Read the model definition and answer for the solid it produces. Units are mm, in the model's axes. A direction names the side the tool comes from. Coordinates: 2 decimals unless noted, no trailing zeros. Loops run counter-clockwise (first coordinate to the right, second up) from the corner with the lowest first, then second, coordinate; pieces in that order, holes last. Notation, with made-up numbers: M 41.25,57.25 L 98.25,57.25 A23 ccw 98.25,72.25 Z; hole C 54,63.25 d8. An arc over 180 degrees is marked long. One line per item, written item: value. Start each with the question number.
1. Flat-ended cylindrical pins translate along their axes: pin 1 (3 mm diameter, centred on x = 15, y = -15.5, fed in from +Z); pin 2 (2 mm diameter, centred on x = 6, y = -37.5, fed in from -Z); pin 3 (8 mm diameter, centred on y = 7.5, z = 14.5, fed in from +X); pin 4 (10 mm diameter, centred on x = 27.5, z = 17, fed in from -Y). Find the tip coordinate at first contact, or state that the pin passes through.
2. The part is cut by section D-D (z = -12). Write down the section's boundary in (x, y).
3. For faces 1 (the face through (-13, -50.8, 7)), 2 (the face through (-0.246, -12.167, 14.285)), determine the directions among +Z, -Z, +X, -X, +Y, -Y from which every point of the face is accessible in a straight line to the end or side of a thin tool.
4. Consider probe 1 along X at (y, z) = (6.5, -13); probe 2 along Z at (x, y) = (48, 21); probe 3 along Z at (x, y) = (18, -45). Determine where each line is inside the solid, lowest interval first.
5. The part is cut by section B-B (x = 0). Write down the section's boundary in (y, z) (1 decimal).
6. Determine the mould class of faces 3 (the face through (22, 25.4, 0)), 4 (the face through (30.824, 12.522, -23.504)), 5 (the face through (-16, -12, 4.762)), 6 (the face through (31.556, 12.522, 23.373)) for opening direction Z: +Z half, -Z half, draft (parallel to the pull), parting line (faces both ways), or undercut.
7. The part is cut by section A-A (y = 9). State how many separate pieces and enclosed holes the cut face has, then the cut area to 3 significant figures.
```python
from build123d import *

# Parameters (mm, degrees)
F0_R     = 14.2875
F1_DEPTH = 25.4
F2_DEPTH = 50.8


with BuildPart() as f1:
    # F0 (on Front) → F1 (new body)
    with BuildSketch(Plane.XZ):
        with BuildLine():
            ThreePointArc((5.042647, -28.126541), (21.916025, -18.336262), (28.575, 0))
            ThreePointArc((28.575, 0), (21.916025, 18.336262), (5.042647, 28.126541))
            ThreePointArc((5.042647, 28.126541), (-28.575, 0), (5.042647, -28.126541))
        make_face()
        with BuildLine():
            ThreePointArc((-13.470384, 4.7625), (0, 14.2875), (13.470384, 4.7625))
            Line((13.470384, 4.7625), (19.05, 4.7625))
            Line((19.05, 4.7625), (19.05, -4.7625))
            Line((19.05, -4.7625), (13.470384, -4.7625))
            ThreePointArc((13.470384, -4.7625), (0, -14.2875), (-13.470384, -4.7625))
            Line((-13.470384, -4.7625), (-19.05, -4.7625))
            Line((-19.05, -4.7625), (-19.05, 4.7625))
            Line((-19.05, 4.7625), (-13.470384, 4.7625))
        make_face(mode=Mode.SUBTRACT)
        with BuildLine():
            ThreePointArc((5.042647, 28.126541), (21.916025, 18.336262), (28.575, 0))
            ThreePointArc((28.575, 0), (21.916025, -18.336262), (5.042647, -28.126541))
            Line((5.042647, -28.126541), (57.336765, -18.751028))
            ThreePointArc((57.336765, -18.751028), (34.925, 0), (57.336765, 18.751028))
            Line((57.336765, 18.751028), (5.042647, 28.126541))
        make_face()
        with BuildLine():
            ThreePointArc((73.025, 0), (68.585683, 12.224174), (57.336765, 18.751028))
            ThreePointArc((57.336765, 18.751028), (34.925, 0), (57.336765, -18.751028))
            ThreePointArc((57.336765, -18.751028), (68.585683, -12.224174), (73.025, 0))
        make_face()
        with Locations((53.975, 0)):
            Circle(F0_R, mode=Mode.SUBTRACT)
    extrude(amount=-F1_DEPTH)

    # F0 (on Front) → F2 (join)
    with BuildSketch(Plane.XZ):
        with BuildLine():
            ThreePointArc((5.042647, -28.126541), (21.916025, -18.336262), (28.575, 0))
            ThreePointArc((28.575, 0), (21.916025, 18.336262), (5.042647, 28.126541))
            ThreePointArc((5.042647, 28.126541), (-28.575, 0), (5.042647, -28.126541))
        make_face()
        with BuildLine():
            ThreePointArc((-13.470384, 4.7625), (0, 14.2875), (13.470384, 4.7625))
            Line((13.470384, 4.7625), (19.05, 4.7625))
            Line((19.05, 4.7625), (19.05, -4.7625))
            Line((19.05, -4.7625), (13.470384, -4.7625))
            ThreePointArc((13.470384, -4.7625), (0, -14.2875), (-13.470384, -4.7625))
            Line((-13.470384, -4.7625), (-19.05, -4.7625))
            Line((-19.05, -4.7625), (-19.05, 4.7625))
            Line((-19.05, 4.7625), (-13.470384, 4.7625))
        make_face(mode=Mode.SUBTRACT)
    extrude(amount=F2_DEPTH)


solid = f1.part
```
Answer block:
1. pin 1: stops at z = 25.18
1. pin 2: stops at z = -28.13
1. pin 3: stops at x = 69.87
1. pin 4: stops at y = -50.8
2. outline: M -25.93,-50.8 L -7.75,-50.8 L -7.75,25.4 L -25.93,25.4 Z; M 7.75,-50.8 L 25.93,-50.8 L 25.93,0 L 46.22,0 L 46.22,25.4 L 7.75,25.4 Z; M 61.73,0 L 68.77,0 L 68.77,25.4 L 61.73,25.4 Z
3. face 1: +Z, -Z, +X, -X, -Y
3. face 2: +Y, -Y
4. probe 1: x = -25.45 to -5.93, 5.93 to 48.05, 59.9 to 67.9
4. probe 2: z = -20.42 to -12.98, 12.98 to 20.42
4. probe 3: z = -22.19 to -4.76, 4.76 to 22.19
5. outline: M -50.8,-28.6 L 25.4,-28.6 L 25.4,-14.3 L -50.8,-14.3 Z; M -50.8,14.3 L 25.4,14.3 L 25.4,28.6 L -50.8,28.6 Z
6. face 3: draft
6. face 4: -Z half
6. face 5: undercut
6. face 6: +Z half
7. separate pieces: 1
7. enclosed holes: 2
7. area: 3,080 mm2
